```python
from build123d import *

# Parameters (mm, degrees)
C_EXT_HEX_REACH = 9.611
SKETCH2_R       = 3.793174209


with BuildPart() as part:
    # Sketch1 → Revolve1 (revolve)
    with BuildSketch(Plane(origin=(0, 0, 0), x_dir=(0, -1, 0), z_dir=(1, 0, 0)), mode=Mode.PRIVATE) as revolve1_sk:
        with BuildLine():
            Line((2.273224716, 0), (3.182239192, 0))
            Line((3.182239192, 0), (3.666174188, 0.2794))
            Line((3.666174188, 0.2794), (3.666174188, 3.789511232))
            Line((3.666174188, 3.789511232), (4.116605118, 4.239942163))
            ThreePointArc((4.116605118, 4.239942163), (4.171665397, 4.322345693), (4.190999996, 4.419547285))
            Line((4.190999996, 4.419547285), (4.190999996, 4.521147285))
            ThreePointArc((4.190999996, 4.521147285), (4.116605118, 4.700752408), (3.936999996, 4.775147285))
            Line((3.936999996, 4.775147285), (2.197152715, 4.775147285))
            Line((2.197152715, 4.775147285), (2.0193, 4.521147285))
            Line((2.0193, 4.521147285), (2.0193, 0.1778))
            Line((2.0193, 0.1778), (2.273224716, 0))
        make_face()
    revolve(revolve1_sk.sketch.rotate(Axis((0, 0, 0), (0, 0, -1)), 270), axis=Axis((0, 0, 0), (0, 0, -1)))

    # C-Ext Hex: up to this cone (the profile starts outside it)
    c_ext_hex_end = Plane(origin=(0, 0, 0), z_dir=(0, 0, -1)).offset(0.123338045) * Cone(1e-06, 9.987662955, 9.987661955, align=(Align.CENTER, Align.CENTER, Align.MIN), mode=Mode.PRIVATE)
    # Sketch2 → C-Ext Hex (cut, up to the surface)
    with BuildSketch(Plane.XY, mode=Mode.PRIVATE) as c_ext_hex_sk1:
        Circle(SKETCH2_R)
        Polygon((0, 3.666174209), (-3.175, 1.833087105), (-3.175, -1.833087105), (0, -3.666174209), (3.175, -1.833087105), (3.175, 1.833087105), align=None, mode=Mode.SUBTRACT)
    c_ext_hex_tool1 = extrude(c_ext_hex_sk1.sketch, amount=-C_EXT_HEX_REACH, mode=Mode.PRIVATE) - c_ext_hex_end
    add(c_ext_hex_tool1.solids().sort_by_distance((-3.685887, 0, 0))[0], mode=Mode.SUBTRACT)


solid = part.part
```
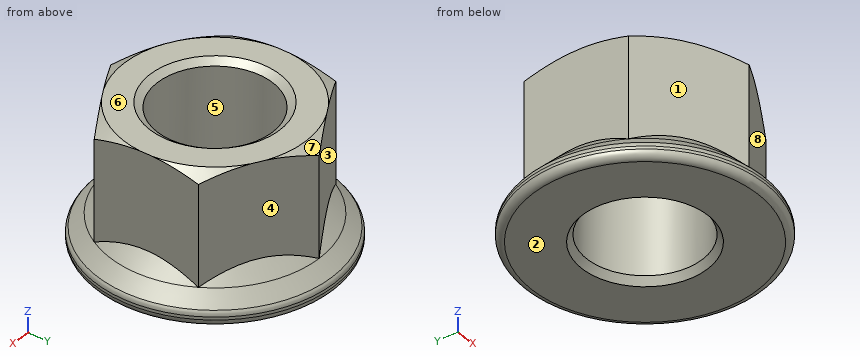
Geometry check sheet. Reference: the model listing, model coordinates, mm. Face numbers are marked on the shaded views. A direction names the side the tool comes from. Give positions to 0.01 mm unless a question says otherwise; leave off trailing zeros. Order: outer loops, then holes, each group sorted by start corner. A loop starts at its lowest first (then second) coordinate and runs counter-clockwise, first axis right, second up. Notation, with made-up numbers: (-19.5, 10) - (39.5, 10) arc R13 ccw to (39.5, 18) - close; hole circle Ø10 at (14, 40.5). An arc over 180 degrees is marked (long way). Answer in a Markdown table with one row per item. Add a question column.
Q1. Material ranges on probe 1 along Y at (x, z) = (-0.5, -2.55); probe 2 along Y at (x, z) = (-1, -3.5); probe 3 along X at (y, z) = (0.75, -0.5) (3 decimals), recorded low to high. Write a range as from..to.
Q2. Cross-section at B-B, the plane z = -3.95. Enter the section's corners in (x, y), then the cut area to 3 significant figures.
Q3. Tool access check on the marked faces 1, 2, 3 and 4. Record the directions out of +Z, -Z, +X, -X, +Y, -Y that give a thin tool (end or side, any length) a straight path to the whole face; none if there is none.
Q4. Cross-section at A-A, the plane z = -0.8. Enter the section's corners in (x, y) (3 decimals), then the cut area to 3 significant figures.
Q5. Gauge pin test, flat ends, axial feed: pin 1 (1.8 mm diameter, centred on y = 0.5, z = -1.5, fed in from -X) (3 decimals); pin 2 (1 mm diameter, centred on x = -3, y = 3, fed in from +Z); pin 3 (1.8 mm diameter, centred on y = -0.5, z = -2, fed in from +X) (3 decimals); pin 4 (3.5 mm diameter, centred on x = 0, y = 0, fed in from -Z). Record the tip position at first contact, or that the pin passes through.
Q6. Mould release check, pull along X, two halves, no side actions. Record for the marked faces 5, 6, 7 and 8: pulls with the +X half, pulls with the -X half, needs draft (parallel to the pull), parting line crosses it, or undercut.
Check values:
| question | item | result |
|---|---|---|
| 1 | probe 1 | y = -3.38..-1.96, 1.96..3.38 |
| 1 | probe 2 | y = -3.23..-1.75, 1.75..3.23 |
| 1 | probe 3 | x = -3.175..-1.875, 1.875..3.175 |
| 2 | outline | circle Ø7.65 at (0, 0); hole circle Ø4.04 at (0, 0) |
| 2 | area | 33.2 mm^2 |
| 3 | face 1 | +Z, -X, -Y |
| 3 | face 2 | -Z, +X, -X, +Y, -Y |
| 3 | face 3 | +Z, -X, +Y |
| 3 | face 4 | +Z, +X, +Y |
| 4 | outline | (-3.175, -1.833) - (0, -3.666) - (3.175, -1.833) - (3.175, 1.833) - (0, 3.666) - (-3.175, 1.833) - close; hole circle Ø4.039 at (0, 0) |
| 4 | area | 22.1 mm^2 |
| 5 | pin 1 | stops at x = -3.175 |
| 5 | pin 2 | stops at z = -3.87 |
| 5 | pin 3 | stops at x = 3.175 |
| 5 | pin 4 | passes through |
| 6 | face 5 | undercut |
| 6 | face 6 | needs draft |
| 6 | face 7 | parting line crosses it |
| 6 | face 8 | pulls with the +X half |
